```python
from build123d import *

# Parameters (mm, degrees)
SKETCH1_W           = 80
SKETCH1_H           = 40
BOSS_EXTRUDE2_DEPTH = 6
CUT_EXTRUDE3_REACH  = 8
SKETCH1_3_R         = 2.555


with BuildPart() as part:
    # Sketch1 → Boss-Extrude2 (new body)
    with BuildSketch(Plane.YZ):
        Rectangle(SKETCH1_W, SKETCH1_H)
    extrude(amount=BOSS_EXTRUDE2_DEPTH)

    # Sketch1_3 → Cut-Extrude3 (cut, up to next)
    with BuildSketch(Plane.YZ, mode=Mode.PRIVATE) as cut_extrude3_sk1:
        with Locations((-25, -4.29)):
            Circle(SKETCH1_3_R)
    cut_extrude3_tool1 = extrude(cut_extrude3_sk1.sketch, amount=CUT_EXTRUDE3_REACH, mode=Mode.PRIVATE) & part.part
    add(cut_extrude3_tool1.solids().sort_by_distance((0, -25, -4.29))[0], mode=Mode.SUBTRACT)
    # Sketch1_3 → Cut-Extrude3 (cut, up to next)
    with BuildSketch(Plane.YZ, mode=Mode.PRIVATE) as cut_extrude3_sk2:
        with Locations((25.8, -4.29)):
            Circle(SKETCH1_3_R)
    cut_extrude3_tool2 = extrude(cut_extrude3_sk2.sketch, amount=CUT_EXTRUDE3_REACH, mode=Mode.PRIVATE) & part.part
    add(cut_extrude3_tool2.solids().sort_by_distance((0, 25.8, -4.29))[0], mode=Mode.SUBTRACT)
    # Sketch1_3 → Cut-Extrude3 (cut, up to next)
    with BuildSketch(Plane.YZ, mode=Mode.PRIVATE) as cut_extrude3_sk3:
        with Locations((-25, 10)):
            Circle(SKETCH1_3_R)
    cut_extrude3_tool3 = extrude(cut_extrude3_sk3.sketch, amount=CUT_EXTRUDE3_REACH, mode=Mode.PRIVATE) & part.part
    add(cut_extrude3_tool3.solids().sort_by_distance((0, -25, 10))[0], mode=Mode.SUBTRACT)
    # Sketch1_3 → Cut-Extrude3 (cut, up to next)
    with BuildSketch(Plane.YZ, mode=Mode.PRIVATE) as cut_extrude3_sk4:
        with Locations((25, 10)):
            Circle(SKETCH1_3_R)
    cut_extrude3_tool4 = extrude(cut_extrude3_sk4.sketch, amount=CUT_EXTRUDE3_REACH, mode=Mode.PRIVATE) & part.part
    add(cut_extrude3_tool4.solids().sort_by_distance((0, 25, 10))[0], mode=Mode.SUBTRACT)


solid = part.part
```
The model under review builds one solid part; all positions refer to its coordinate system, in mm. Round coordinates to 2 decimals unless told otherwise and drop trailing zeros. Loops run counter-clockwise (first coordinate to the right, second up) from the corner with the lowest first, then second, coordinate; pieces in that order, holes last. Notation, with made-up numbers: (10.25, 39.25) - (15.25, 39.25) arc R29 ccw to (15.25, 70.25) - close; hole circle Ø2 at (5.25, -7.5). An arc over 180 degrees is marked (long way). Write each question's results on one line, items separated by ' | '. Start each with the question number.
Q1. Take a section at B-B on x = 1.65. Give the boundary of the cut face in (y, z) (3 decimals).
Q2. Take a section at A-A on z = 10. Give the boundary of the cut face in (x, y) (3 decimals), plus the area to 3 significant figures.
Q3. Wall thickness on line 1 along Y through (x, z) = (4.3, -4.29) (3 decimals); line 2 along Y through (x, z) = (1.4, 10) (3 decimals); line 3 along Z through (x, y) = (2.2, -25) (3 decimals): over which ranges is each line inside the solid? List them lowest first. Write a range as [from, to].
Q4. Take a section at C-C on y = 25.8. Give the boundary of the cut face in (x, z) (3 decimals).
Q5. Draft analysis for pull direction Z (two halves, no side actions). For faces 1 (the flat face through (3, -1, 20)), 2 (the cylindrical face through (2.958, 23.247, -4.178)), 3 (the flat face through (6, -1, 0)), state which applies: pulls with the +Z half, pulls with the -Z half, needs draft (parallel to the pull), parting line crosses it, or undercut.
Data:
1) outline: (-40, -20) - (40, -20) - (40, 20) - (-40, 20) - close; hole circle Ø5.11 at (-25, -4.29); hole circle Ø5.11 at (-25, 10); hole circle Ø5.11 at (25, 10); hole circle Ø5.11 at (25.8, -4.29)
2) outline: (0, -40) - (6, -40) - (6, -27.555) - (0, -27.555) - close; (0, -22.445) - (6, -22.445) - (6, 22.445) - (0, 22.445) - close; (0, 27.555) - (6, 27.555) - (6, 40) - (0, 40) - close | area: 419 mm²
3) line 1: y = [-40, -27.555], [-22.445, 23.245], [28.355, 40] | line 2: y = [-40, -27.555], [-22.445, 22.445], [27.555, 40] | line 3: z = [-20, -6.845], [-1.735, 7.445], [12.555, 20]
4) outline: (0, -20) - (6, -20) - (6, -6.845) - (0, -6.845) - close; (0, -1.735) - (6, -1.735) - (6, 7.573) - (0, 7.573) - close; (0, 12.427) - (6, 12.427) - (6, 20) - (0, 20) - close
5) face 1: pulls with the +Z half | face 2: undercut | face 3: needs draft
